Work out the finished part from the listing and answer in its coordinate system (mm). Round coordinates to 2 decimals unless told otherwise and drop trailing zeros. Order: outer loops, then holes, each group sorted by start corner. A loop starts at its lowest first (then second) coordinate and runs counter-clockwise, first axis right, second up. Notation, with made-up numbers: (46, 29.25) -> (84, 29.25) arc R19 cw to (84, 63.25) -> close; hole circle Ø9 at (67, 89.5). An arc over 180 degrees is marked (long way). Use a Markdown table: item, result. Add a question column.
Item 1: A cutting plane is placed at D-D, the plane x = 118. Determine the outline of the cut face in (y, z) (3 decimals).
Item 2: A cutting plane is placed at A-A, the plane x = -14.5. Determine the outline of the cut face in (y, z) (3 decimals).
Item 3: A cutting plane is placed at B-B, the plane z = -0.6. Determine the outline of the cut face in (x, y) (3 decimals), plus the area to 3 significant figures.
Item 4: A cutting plane is placed at C-C, the plane y = -466. Determine the outline of the cut face in (x, z) (3 decimals).
Item 5: Find the intervals of material crossed by L1, parallel to Y at x = 50.5, z = -1.95; L2, parallel to Y at x = 111, z = -2.5; L3, parallel to Y at x = -20.5, z = -2.8, in increasing order. Write a range as [from, to].
Item 6: Flat-ended cylindrical pins translate along their axes: P1, Ø8.5, axis at x = -64.71, y = -437.72, coming from the +Z side; P2, Ø1, axis at y = -443.5, z = -2, coming from the +X side; P3, Ø1, axis at x = -50, z = -2, coming from the +Y side; P4, Ø1.6, axis at x = 142.5, z = -1.5, coming from the -Y side. Find the tip coordinate at first contact, or state that the pin passes through.
Autodesk Inventor part; units mm, degrees
ref_plane "YZ Plane" through (0, 0, 0) normal (1, 0, 0) x (0, 1, 0)
ref_plane "XZ Plane" through (0, 0, 0) normal (0, 1, 0) x (-1, 0, 0)
ref_plane "XY Plane" through (0, 0, 0) normal (0, 0, 1) x (1, 0, 0)
sketch "Sketch1" plane through (0, 0, 0) normal (0, 0, 1) x (1, 0, 0)
  line L0 (176.5882, -640.9214) -> (176.5882, 349.6786)
  line L1 (-77.4118, 349.6786) -> (-77.4118, -640.9214)
  line L2 (100.3882, -640.9214) -> (100.3882, -564.7214)
  line L3 (100.3882, -564.7214) -> (176.5882, -564.7214)
  line L4 (176.5882, -475.8214) -> (100.3882, -475.8214)
  line L5 (100.3882, -475.8214) -> (100.3882, -399.6214)
  line L6 (100.3882, -399.6214) -> (176.5882, -399.6214)
  line L7 (176.5882, -399.6214) -> (176.5882, -475.8214)
  line L8 (176.5882, -94.8214) -> (100.3882, -94.8214)
  line L9 (176.5882, 70.2786) -> (176.5882, -94.8214)
  line L10 (-77.4118, 8.6504) -> (-77.4118, 88.2844)
  line L11 (-77.4118, -379.8866) -> (-77.4118, -294.668)
  line L12 (-77.4118, -640.9214) -> (-1.2118, -640.9214)
  line L13 (-1.2118, -640.9214) -> (-1.2118, -564.7214)
  line L14 (-1.2118, -564.7214) -> (-77.4118, -564.7214)
  line L15 (-77.4118, -564.7214) -> (-77.4118, -640.9214)
  line L16 (-77.4118, -259.9214) -> (-1.2118, -259.9214)
  line L17 (-1.2118, -259.9214) -> (-1.2118, -336.1214)
  line L18 (-1.2118, -336.1214) -> (-77.4118, -336.1214)
  line L19 (-77.4118, -336.1214) -> (-77.4118, -259.9214)
  line L20 (-1.2118, -82.1214) -> (-1.2118, 19.4786)
  line L21 (-77.4118, 19.4786) -> (-77.4118, 19.4786)
  line L22 (100.3882, -640.9214) -> (100.3882, -666.3214)
  line L23 (100.3882, -666.3214) -> (-1.2118, -666.3214)
  line L24 (-1.2118, -666.3214) -> (-1.2118, -640.9214)
  line L25 (-1.2118, -82.1214) -> (-77.4118, -82.1214)
  line L26 (100.3882, 19.4786) -> (100.3882, -94.8214)
  line L27 (100.3882, 19.4786) -> (-1.2118, 19.4786)
  point P0 (0, 0)
  point P1 (49.5882, -323.4214)
  point P2 (-64.7118, -437.7214)
  point P3 (-64.7118, -132.9214)
  point P4 (163.8882, -196.4214)
  point P5 (163.8882, -513.9214)
  point P6 (49.5882, -653.6214)
  point P7 (49.5882, 6.7786)
  dimension "d1" = 990.6
  dimension "d2" = 76.2
  dimension "d3" = 76.2
  dimension "d4" = 76.2
  dimension "d5" = 76.2
  dimension "d6" = 88.9
  dimension "d7" = 304.8
  dimension "d14" = 76.2
  dimension "d15" = 76.2
  dimension "d16" = 76.2
  dimension "d17" = 76.2
  dimension "d18" = 63.5
  dimension "d19" = 101.6
  dimension "d20" = 76.2
  dimension "d29" = 12.7
  dimension "d30" = 12.7
  dimension "d31" = 127
  dimension "d32" = 101.6
  dimension "d33" = 12.7
  dimension "d34" = 12.7
  dimension "d35" = 101.6
  dimension "d36" = 38.1
  dimension "d37" = 25.4
  dimension "d38" = 101.6
  dimension "d49" = 101.6
  dimension "d50" = 114.3
  dimension "d51" = 76.2
  dimension "d52" = 76.2
extrude "Extrusion1" add sketch "Sketch1" against normal blind 3.175 contours L3 L2 L22 L23 L24 L13 L14 L1 L18 L17 L16 L25 L20 L27 L26 L8 L0 L6 L5 L4
hole "Hole1" at (49.5882, -323.4214, 0) at (-64.7118, -437.7214, 0) at (-64.7118, -132.9214, 0) at (163.8882, -196.4214, 0) at (163.8882, -513.9214, 0) at (49.5882, -653.6214, 0) at (49.5882, 6.7786, 0) direction (0, 0, -1) diameter 6.35 depth 25.4 tip angle 118
properties part number "medium tower walls"
Reported:
| question | item | result |
|---|---|---|
| 1 | outline | (-564.721, -3.175) -> (-475.821, -3.175) -> (-475.821, 0) -> (-564.721, 0) -> close; (-399.621, -3.175) -> (-94.821, -3.175) -> (-94.821, 0) -> (-399.621, 0) -> close |
| 2 | outline | (-564.721, -3.175) -> (-336.121, -3.175) -> (-336.121, 0) -> (-564.721, 0) -> close; (-259.921, -3.175) -> (-82.121, -3.175) -> (-82.121, 0) -> (-259.921, 0) -> close |
| 3 | outline | (-77.412, -564.721) -> (-1.212, -564.721) -> (-1.212, -666.321) -> (100.388, -666.321) -> (100.388, -564.721) -> (176.588, -564.721) -> (176.588, -475.821) -> (100.388, -475.821) -> (100.388, -399.621) -> (176.588, -399.621) -> (176.588, -94.821) -> (100.388, -94.821) -> (100.388, 19.479) -> (-1.212, 19.479) -> (-1.212, -82.121) -> (-77.412, -82.121) -> (-77.412, -259.921) -> (-1.212, -259.921) -> (-1.212, -336.121) -> (-77.412, -336.121) -> close; hole circle Ø6.35 at (-64.712, -437.721); hole circle Ø6.35 at (-64.712, -132.921); hole circle Ø6.35 at (49.588, -653.621); hole circle Ø6.35 at (49.588, -323.421); hole circle Ø6.35 at (49.588, 6.779); hole circle Ø6.35 at (163.888, -513.921); hole circle Ø6.35 at (163.888, -196.421) |
| 3 | area | 130,000 mm² |
| 4 | outline | (-77.412, -3.175) -> (100.388, -3.175) -> (100.388, 0) -> (-77.412, 0) -> close |
| 5 | L1 | [-666.32, -656.66], [-650.58, -326.46], [-320.38, 3.74], [9.82, 19.48] |
| 5 | L2 | [-564.72, -475.82], [-399.62, -94.82] |
| 5 | L3 | [-564.72, -336.12], [-259.92, -82.12] |
| 6 | P1 | z = 0 |
| 6 | P2 | x = 100.39 |
| 6 | P3 | y = -82.12 |
| 6 | P4 | y = -564.72 |
